from build123d import *
from OCP.BRepFilletAPI import BRepFilletAPI_MakeChamfer

# Parameters (mm, degrees)
SKETCH1_R           = 6
BOSS_EXTRUDE1_DEPTH = 5
SKETCH2_R           = 1.6
CUT_EXTRUDE1_DEPTH  = 25
CHAMFER1_SIZE       = 10
CHAMFER1_SIZE2      = 10.246835966
CHAMFER2_SIZE       = 10
CHAMFER2_SIZE2      = 11.000628676


with BuildPart() as part:
    # Sketch1 → Boss-Extrude1 (new body)
    with BuildSketch(Plane.XY):
        with BuildLine():
            Line((80, 30), (-80, 30))
            Line((-80, 30), (-87.408238134, 114.676549338))
            Line((-87.408238134, 114.676549338), (-116.370756775, 112.836156983))
            Line((-116.370756775, 112.836156983), (-129.776384549, 3.656080302))
            ThreePointArc((-129.776384549, 3.656080302), (-122.468671624, -19.878601446), (-100, -30))
            Line((-100, -30), (100, -30))
            ThreePointArc((100, -30), (122.468671624, -19.878601446), (129.776384549, 3.656080302))
            Line((129.776384549, 3.656080302), (116.370756775, 112.836156983))
            Line((116.370756775, 112.836156983), (87.408238134, 114.676549338))
            Line((87.408238134, 114.676549338), (80, 30))
        make_face()
        with Locations((-100, 0)):
            Circle(SKETCH1_R, mode=Mode.SUBTRACT)
        with Locations((100, 0)):
            Circle(SKETCH1_R, mode=Mode.SUBTRACT)
    extrude(amount=BOSS_EXTRUDE1_DEPTH)

    # Sketch2 → Cut-Extrude1 (cut)
    with BuildSketch(Plane(origin=(0, 0, 0), x_dir=(-1, 0, 0), z_dir=(0, 0, -1))):
        with Locations((109, 98.696293654)):
            Circle(SKETCH2_R)
        with Locations((-109, 98.696293654)):
            Circle(SKETCH2_R)
        Polygon((120.438781703, 79.704752691), (110.79653452, 88.696293654), (114.490425578, 104.696293654), (117.165001342, 106.367554078), align=None)
        Polygon((-117.165001342, 106.367554078), (-120.438781703, 79.704752691), (-110.79653452, 88.696293654), (-114.490425578, 104.696293654), align=None)
    extrude(amount=-CUT_EXTRUDE1_DEPTH, mode=Mode.SUBTRACT)

    # Chamfer1: one chamfer whose edges measure the first distance from different faces: ONE call of the kernel's chamfer builder (chamfer() names one face for all edges)
    chamfer1_edges_1 = [part.edges().sort_by_distance(p)[0] for p in [
        (-87.408238134, 114.676549338, 2.5),
    ]]
    chamfer1_side_1 = [part.faces().sort_by_distance(p)[0] for p in [
        (-83.704119067, 72.338274669, 2.5),
    ]]
    chamfer1_edges_2 = [part.edges().sort_by_distance(p)[0] for p in [
        (87.408238134, 114.676549338, 2.5),
    ]]
    chamfer1_side_2 = [part.faces().sort_by_distance(p)[0] for p in [
        (101.889497454, 113.75635316, 2.5),
    ]]
    chamfer1 = BRepFilletAPI_MakeChamfer(part.part.solid().wrapped)
    for e in chamfer1_edges_1:
        chamfer1.Add(CHAMFER1_SIZE, CHAMFER1_SIZE2, e.wrapped, chamfer1_side_1[0].wrapped)  # the first distance lies on this face
    for e in chamfer1_edges_2:
        chamfer1.Add(CHAMFER1_SIZE, CHAMFER1_SIZE2, e.wrapped, chamfer1_side_2[0].wrapped)  # the first distance lies on this face
    add(Compound.cast(chamfer1.Shape()), mode=Mode.REPLACE)

    # Chamfer2: one chamfer whose edges measure the first distance from different faces: ONE call of the kernel's chamfer builder (chamfer() names one face for all edges)
    chamfer2_edges_1 = [part.edges().sort_by_distance(p)[0] for p in [
        (-80, 30, 2.5),
    ]]
    chamfer2_side_1 = [part.faces().sort_by_distance(p)[0] for p in [
        (0, 30, 2.5),
    ]]
    chamfer2_edges_2 = [part.edges().sort_by_distance(p)[0] for p in [
        (80, 30, 2.5),
    ]]
    chamfer2_side_2 = [part.faces().sort_by_distance(p)[0] for p in [
        (83.257583767, 67.234352838, 2.5),
    ]]
    chamfer2 = BRepFilletAPI_MakeChamfer(part.part.solid().wrapped)
    for e in chamfer2_edges_1:
        chamfer2.Add(CHAMFER2_SIZE, CHAMFER2_SIZE2, e.wrapped, chamfer2_side_1[0].wrapped)  # the first distance lies on this face
    for e in chamfer2_edges_2:
        chamfer2.Add(CHAMFER2_SIZE, CHAMFER2_SIZE2, e.wrapped, chamfer2_side_2[0].wrapped)  # the first distance lies on this face
    add(Compound.cast(chamfer2.Shape()), mode=Mode.REPLACE)


solid = part.part
Part model, mm, in its own coordinate system. A direction names the side the tool comes from. Coordinates: 2 decimals unless noted, no trailing zeros. Loops run counter-clockwise (first coordinate to the right, second up) from the corner with the lowest first, then second, coordinate; pieces in that order, holes last. Notation, with made-up numbers: M 12,66.25 L 34,66.25 A34 ccw 34,97.25 Z; hole C -19.5,-10 d3. An arc over 180 degrees is marked long. Use a Markdown table: item, result. Add a question column.
Q1. Cut at B-B (y = 93). Write the cut outline in (x, z), and give its area (3 significant figures).
Q2. Cut at A-A (y = 0). Write the cut outline in (x, z), and give its area (3 significant figures).
Q3. Mould opens along X. For faces 1 (the flat face through (-115.685, 84.138, 2.465)), 2 (the flat face through (115.685, 84.138, 2.465)), 3 (the flat face through (91.88, 109.19, 2.47)) say: +X half, -X half, draft (parallel to the pull), parting line (faces both ways), or undercut.
Q4. Which spindle directions (+Z, -Z, +X, -X, +Y, -Y) get a long thin tool onto all of the face, cutting with end or side? Do faces 4 (the cylindrical face through (94, 0, 2)), 5 (the flat face through (83.733, 72.667, 2.465)), 6 (the flat face through (112.618, 96.584, 2.465)), 7 (the flat face through (-112.618, 96.584, 2.465)). Say none if no direction does.
Q5. Probe L1, parallel to X at y = -2, z = 3.1; L2, parallel to Y at x = 2, z = 4.6; L3, parallel to X at y = 94, z = 1.95. List the from-to ranges inside material, lowest first.
Q6. Cut at D-D (x = 16). Write the cut outline in (y, z), and give its area (3 significant figures).
Q7. Cut at C-C (z = 2.95). Write the cut outline in (x, y) (3 decimals).
Q8. Pin check, flat tips, straight feed: P1, Ø1.5, axis at y = 42, z = 4, coming from the +X side; P2, Ø1, axis at y = 33.5, z = 3, coming from the +X side; P3, Ø1.5, axis at x = 10, z = 3.5, coming from the +Y side. Stop position of each tip, or through.
Worked out:
| question | item | result |
|---|---|---|
| 1 | outline | M -111.79,0 L -85.51,0 L -85.51,5 L -111.79,5 Z; M 85.51,0 L 111.79,0 L 111.79,5 L 85.51,5 Z |
| 1 | area | 263 mm2 |
| 2 | outline | M -130,0 L -106,0 L -106,5 L -130,5 Z; M -94,0 L 94,0 L 94,5 L -94,5 Z; M 106,0 L 130,0 L 130,5 L 106,5 Z |
| 2 | area | 1,180 mm2 |
| 3 | face 1 | -X half |
| 3 | face 2 | +X half |
| 3 | face 3 | undercut |
| 4 | face 4 | +Z, -Z |
| 4 | face 5 | +Z, -Z, +Y |
| 4 | face 6 | +Z, -Z, +X |
| 4 | face 7 | +Z, -Z, -X |
| 5 | L1 | x = -129.93 to -105.66, -94.34 to 94.34, 105.66 to 129.93 |
| 5 | L2 | y = -30 to 30 |
| 5 | L3 | x = -112.02 to -85.6, 85.6 to 112.02 |
| 6 | outline | M -30,0 L 30,0 L 30,5 L -30,5 Z |
| 6 | area | 300 mm2 |
| 7 | outline | M -129.776,3.656 A30 ccw -100,-30 L 100,-30 A30 ccw 129.776,3.656 L 120.439,79.705 L 110.797,88.696 L 114.49,104.696 L 117.165,106.368 L 116.371,112.836 L 97.388,114.042 L 86.515,104.469 L 80.872,39.962 L 68.999,30 L -70,30 L -80.959,40.959 L -86.537,104.715 L -97.634,114.027 L -116.371,112.836 L -117.165,106.368 L -114.49,104.696 L -110.797,88.696 L -120.439,79.705 Z; hole C -109,98.696 d3.2; hole C -100,0 d12; hole C 100,0 d12; hole C 109,98.696 d3.2 |
| 8 | P1 | stops at x = 125.16 |
| 8 | P2 | stops at x = 126.17 |
| 8 | P3 | stops at y = 30 |
